from build123d import *

# Parameters (mm, degrees)
F0_W     = 15
F0_H     = 10.6
F0_R     = 2.3
F1_DEPTH = 2
F2_DEPTH = 8
F3_W     = 8.5
F3_H     = 3
F4_DEPTH = 9
F5_START = 7
F3_H_2   = 1.5
F5_DEPTH = 2


# Not quite as in the source:
# - a feature names something its author has since deleted; it is built from what else it names


with BuildPart() as f1:
    # F0 (on Top) → F1 (new body)
    with BuildSketch(Plane.XY):
        with Locations((-7.5, 0)):
            Rectangle(F0_W, F0_H)
        with Locations((-7.5, 0)):
            Circle(F0_R, mode=Mode.SUBTRACT)
        with Locations((7.5, 0)):
            Rectangle(F0_W, F0_H)
        with Locations((7.5, 0)):
            Circle(F0_R, mode=Mode.SUBTRACT)
    extrude(amount=-F1_DEPTH)

    # F0 (on Top) → F2 (join)
    with BuildSketch(Plane.XY):
        with Locations((-7.5, 0)):
            Circle(F0_R)
        with Locations((7.5, 0)):
            Circle(F0_R)
    extrude(amount=-F2_DEPTH)

    # F3 (on Top) → F4 (join)
    with BuildSketch(Plane.XY):
        with Locations((0, -1.5)):
            Rectangle(F3_W, F3_H)
    extrude(amount=F4_DEPTH)

    # F3 (on Top) → F5 (join)
    with BuildSketch(Plane.XY.offset(F5_START)):
        with Locations((0, 0.75)):
            Rectangle(F3_W, F3_H_2)
    extrude(amount=F5_DEPTH)


solid = f1.part
Read the model definition and answer for the solid it produces. Units are mm, in the model's axes. A direction names the side the tool comes from. Give positions to 0.01 mm unless a question says otherwise; leave off trailing zeros. Write each loop counter-clockwise with the first axis right and the second up, starting at its lowest first coordinate (ties: lowest second). Pieces come first, ordered by that corner, then holes. Notation, with made-up numbers: (31.25, -32) - (82.25, -32) arc R5 ccw to (82.25, -26) - close; hole circle Ø7 at (67, 79). An arc over 180 degrees is marked (long way). Return JSON: item names as keys, results as strings.
Q1. For faces 4 (the face through (-9.798, 0.101, -4.958)), 5 (the face through (0, 0, 3)), 6 (the face through (4.25, -1, 4)), determine the directions among +Z, -Z, +X, -X, +Y, -Y from which every point of the face is accessible in a straight line to the end or side of a thin tool.
Reply:
{"face 4": "-Z", "face 5": "+X, -X, +Y", "face 6": "+Z, +X, +Y, -Y"}
Q2. A cutting plane is placed at C-C, the plane y = -1.5. Determine the outline of the cut face in (x, z).
Reply:
{"outline": "(-15, -2) - (-9.24, -2) - (-9.24, -8) - (-5.76, -8) - (-5.76, -2) - (5.76, -2) - (5.76, -8) - (9.24, -8) - (9.24, -2) - (15, -2) - (15, 0) - (4.25, 0) - (4.25, 9) - (-4.25, 9) - (-4.25, 0) - (-15, 0) - close"}
Q3. A cutting plane is placed at B-B, the plane z = -5. Determine the outline of the cut face in (x, y).
Reply:
{"outline": "circle Ø4.6 at (-7.5, 0); circle Ø4.6 at (7.5, 0)"}
Q4. Given P1, Ø2, axis at y = -2, z = 2.5, coming from the +X side; P2, Ø3.5, axis at y = -2, z = 4.5, coming from the -X side; P3, Ø4, axis at x = 2.5, y = -2, coming from the -Z side; P4, Ø4, axis at x = 8, z = 5, coming from the +Y side, each flat-ended and moving along its own axis, determine where each tip first touches the part or whether it passes through.
Reply:
{"P1": "x = 4.25", "P2": "x = -4.25", "P3": "z = -2", "P4": "through"}
Q5. A cutting plane is placed at D-D, the plane z = 4.25. Determine the outline of the cut face in (x, y).
Reply:
{"outline": "(-4.25, -3) - (4.25, -3) - (4.25, 0) - (-4.25, 0) - close"}
Q6. Consider line 1 along Z through (x, y) = (8.5, 1.25); line 2 along Z through (x, y) = (9, -2.75); line 3 along X through (y, z) = (1, -3.5). Determine where each line is inside the solid, lowest interval first. Write a range as [from, to].
Reply:
{"line 1": "[-8, 0]", "line 2": "[-2, 0]", "line 3": "[-9.57, -5.43], [5.43, 9.57]"}
Q7. A cutting plane is placed at A-A, the plane x = 7.5. Determine the outline of the cut face in (y, z).
Reply:
{"outline": "(-5.3, -2) - (-2.3, -2) - (-2.3, -8) - (2.3, -8) - (2.3, -2) - (5.3, -2) - (5.3, 0) - (-5.3, 0) - close"}
Q8. For a pull along X with two mould halves and no side action, classify faces 1 (the face through (-15, 0, -1)), 2 (the face through (-8, 0, -8)), 3 (the face through (0, 0, -2)) as released by +X, released by -X, zero draft, split by the parting line, or undercut.
Reply:
{"face 1": "released by -X", "face 2": "zero draft", "face 3": "undercut"}
